Check sheet for the modelled part. Datum: model origin and axes. Units: mm. A direction names the side the tool comes from. Round coordinates to 2 decimals unless told otherwise and drop trailing zeros. Write each loop counter-clockwise with the first axis right and the second up, starting at its lowest first coordinate (ties: lowest second). Pieces come first, ordered by that corner, then holes. Notation, with made-up numbers: (-10, 24) -> (46, 24) arc R19 cw to (46, 30) -> close; hole circle Ø5 at (-12, -12.75). An arc over 180 degrees is marked (long way). One line per item, written item: value. Start each with the question number.
Autodesk Inventor part; units mm, degrees
ref_plane "YZ Plane" through (0, 0, 0) normal (1, 0, 0) x (0, 1, 0)
ref_plane "XZ Plane" through (0, 0, 0) normal (0, 1, 0) x (-1, 0, 0)
ref_plane "XY Plane" through (0, 0, 0) normal (0, 0, 1) x (1, 0, 0)
sketch "Sketch1" plane through (0, 0, 0) normal (1, 0, 0) x (0, 1, 0)
  line L0 (0, 0) -> (33.25, 0)
  line L1 (33.25, 0) -> (33.25, -33.25)
  line L2 (33.25, -33.25) -> (0, -33.25)
  line L3 (0, -33.25) -> (0, 0)
  dimension "d0" = 33.25
  dimension "d1" = 33.25
extrude "Extrusion1" add sketch "Sketch1" along normal blind 30
sketch "Sketch2" plane through (30, 0, 0) normal (1, 0, 0) x (0, 0, -1)
  line L0 (3.25, 3.25) -> (30, 3.25)
  line L1 (30, 3.25) -> (30, 30)
  line L2 (30, 30) -> (3.25, 30)
  line L3 (3.25, 30) -> (3.25, 3.25)
  point P0 (0, 0)
  dimension "d4" = 26.75
  dimension "d5" = 26.75
sketch "Sketch3" plane through (30, 0, 0) normal (1, 0, 0) x (0, 0, -1)
  line L0 (33.25, 0) -> (33.25, 33.25)
  line L1 (0, 0) -> (33.25, 0)
  line L2 (33.25, 0) -> (33.25, 33.25)
  line L3 (33.25, 33.25) -> (0, 33.25)
  line L4 (0, 33.25) -> (0, 0)
sketch "Sketch4" plane through (30, 0, 0) normal (1, 0, 0) x (0, 0, -1)
  line L0 (3.25, 3.25) -> (30, 3.25)
  line L1 (30, 3.25) -> (30, 30)
  line L2 (30, 30) -> (3.25, 30)
  line L3 (3.25, 30) -> (3.25, 3.25)
  line L4 (0, 33.25) -> (0, 0)
  line L5 (33.25, 0) -> (33.25, 33.25)
  line L6 (0, 0) -> (33.25, 0)
  line L7 (33.25, 0) -> (33.25, 33.25)
  line L8 (33.25, 33.25) -> (0, 33.25)
  line L9 (0, 33.25) -> (0, 0)
  dimension "d6" = 26.75
  dimension "d7" = 26.75
extrude "Extrusion2" cut sketch "Sketch4" against normal blind 3
chamfer "Chamfer1" distance 1.875 angle 45 8 edges at (13.5, 33.25, 0) (13.5, 33.25, -33.25) (28.5, 30, -3.25) (28.5, 30, -30) (28.5, 3.25, -3.25) (13.5, 0, 0) (28.5, 3.25, -30) (13.5, 0, -33.25)
sketch "Sketch5" plane through (30, 0, 0) normal (1, 0, 0) x (0, 0, -1)
  line L0 (9.875, 9.875) -> (23.375, 9.875)
  line L1 (23.375, 9.875) -> (23.375, 23.375)
  line L2 (23.375, 23.375) -> (9.875, 23.375)
  line L3 (9.875, 23.375) -> (9.875, 9.875)
  line L4 (28.125, 30) -> (5.125, 30)
  line L5 (30, 5.125) -> (30, 28.125)
  line L6 (3.25, 3.25) -> (30, 3.25)
  line L7 (30, 3.25) -> (30, 30)
  line L8 (30, 30) -> (3.25, 30)
  line L9 (3.25, 30) -> (3.25, 3.25)
  point P0 (0, 0)
  dimension "d13" = 13.5
  dimension "d14" = 13.5
  dimension "d15" = 6.625
  dimension "d16" = 6.625
extrude "Extrusion3" cut sketch "Sketch5" against normal blind 26.75 contours L3 L2 L1 L0
sketch "Sketch6" plane through (0, 1.875, 0) normal (0, 0, 1) x (1, 0, 0)
  point P0 (0, -1.875)
sketch "Sketch7" plane through (0, 1.875, 0) normal (0, 0, 1) x (1, 0, 0)
  circle A0 centre (18.125, 14.75) radius 4.625
  point P0 (0, -1.875)
  dimension "d19" = 9.25
extrude "Extrusion4" cut sketch "Sketch7" against normal blind 33.25
sketch "Sketch8" plane through (0, 0, -31.375) normal (0, -1, 0) x (1, 0, 0)
  circle A0 centre (18.125, 14.75) radius 4.625
  point P0 (0, 31.375)
  dimension "d22" = 9.25
extrude "Extrusion5" cut sketch "Sketch8" against normal blind 33.25
thread "Thread1"
thread "Thread2"
thread "Thread3"
thread "Thread4"
sketch "Sketch9" plane through (0, 0, 0) normal (-1, 0, 0) x (0, 0, 1)
  circle A0 centre (-16.625, 16.625) radius 4.625
  point P0 (0, 0)
  dimension "d33" = 9.25
extrude "Extrusion6" cut sketch "Sketch9" against normal blind 10
thread "Thread5"
properties part number "cuvette holder blockBASE_with_bottom_drain"
1. Depth check by flat-ended pin: pin 1 Ø3.5 at (x, y) = (28, 12.5) entering from -Z; pin 2 Ø0.9 at (x, y) = (29, 11.5) entering from +Z; pin 3 Ø5.5 at (x, y) = (18.125, 16.625) entering from +Z; pin 4 Ø1.5 at (x, z) = (29, -11.5) entering from -Y. Enter the tip coordinate at first touch or a pass-through.
2. Access from +Z, -Z, +X, -X, +Y, -Y to the whole of each face (thin tool, end or side, straight path). Record for faces 4 (the face through (14, 14, -23.375)), 5 (the face through (29, 3.25, -16)), 6 (the face through (29, 17, -3.25)), 7 (the face through (29, 30, -17)).
3. Material ranges on probe 1 along Y at (x, z) = (5.75, -20.5) (3 decimals); probe 2 along Z at (x, y) = (28.5, 10) (3 decimals); probe 3 along Z at (x, y) = (11.5, 22) (3 decimals), recorded low to high.
4. Cross-section at D-D (x = 20). Record the cut outline in (y, z) (3 decimals), plus the area to 3 significant figures.
5. Release check for a two-part mould opening along X. For faces 1 (the face through (13.689, 0.951, -32.326)), 2 (the face through (0, 13, -13)), 3 (the face through (13.504, 16.828, -4.868)) record: +X half, -X half, draft (parallel to the pull), parting line (faces both ways), or undercut.
6. Cross-section at A-A (x = 9). Record the cut outline in (y, z) (3 decimals), plus the area to 3 significant figures.
7. Cross-section at C-C (y = 6). Record the cut outline in (x, z) (3 decimals).
8. Cross-section at B-B (z = -4). Record the cut outline in (x, y) (3 decimals), plus the area to 3 significant figures.
Working result:
1. pin 1: stops at z = -33.25
1. pin 2: stops at z = -3.25
1. pin 3: passes through
1. pin 4: stops at y = 3.25
2. face 4: +X
2. face 5: +Z, -Z, +X, -Y
2. face 6: +Z, +X, +Y, -Y
2. face 7: +Z, -Z, +X, +Y
3. probe 1: y = 0 to 9.875, 23.375 to 33.25
3. probe 2: z = -30 to -23.375, -9.875 to -3.25
3. probe 3: z = -33.25 to -23.375, -9.875 to 0
4. outline: (0, -31.375) -> (1.875, -33.25) -> (12.397, -33.25) -> (12.397, -23.375) -> (9.875, -23.375) -> (9.875, -20.853) -> (0, -20.853) -> close; (0, -12.397) -> (9.875, -12.397) -> (9.875, -9.875) -> (12.397, -9.875) -> (12.397, 0) -> (1.875, 0) -> (0, -1.875) -> close; (20.853, -33.25) -> (31.375, -33.25) -> (33.25, -31.375) -> (33.25, -20.853) -> (23.375, -20.853) -> (23.375, -23.375) -> (20.853, -23.375) -> close; (20.853, -9.875) -> (23.375, -9.875) -> (23.375, -12.397) -> (33.25, -12.397) -> (33.25, -1.875) -> (31.375, 0) -> (20.853, 0) -> close
4. area: 582 mm^2
5. face 1: draft
5. face 2: -X half
5. face 3: undercut
6. outline: (0, -31.375) -> (1.875, -33.25) -> (31.375, -33.25) -> (33.25, -31.375) -> (33.25, -1.875) -> (31.375, 0) -> (1.875, 0) -> (0, -1.875) -> close; hole (9.875, -23.375) -> (23.375, -23.375) -> (23.375, -9.875) -> (9.875, -9.875) -> close
6. area: 916 mm^2
7. outline: (0, -33.25) -> (27, -33.25) -> (27, -30) -> (30, -30) -> (30, -3.25) -> (27, -3.25) -> (27, 0) -> (0, 0) -> close; hole circle Ø9.25 at (18.125, -16.625)
8. outline: (0, 0) -> (27, 0) -> (27, 4.375) -> (30, 4.375) -> (30, 28.875) -> (27, 28.875) -> (27, 33.25) -> (0, 33.25) -> close; hole circle Ø9.25 at (18.125, 16.625)
8. area: 904 mm^2
